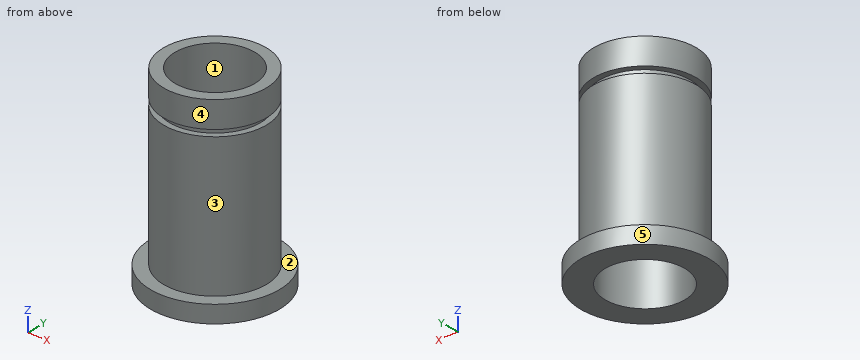
```python
from build123d import *


with BuildPart() as part:
    # Sketch1 → Revolve1 (revolve)
    with BuildSketch(Plane(origin=(0, 0, 0), x_dir=(0, 0, -1), z_dir=(1, 0, 0)), mode=Mode.PRIVATE) as revolve1_sk:
        Polygon((0, 5.9182), (3.048, 5.9182), (3.048, 5.2324), (3.7846, 5.2324), (3.7846, 5.9182), (20, 5.9182), (20, 7.4182), (22, 7.4182), (22, 4.6), (0, 4.6), align=None)
    revolve(revolve1_sk.sketch.rotate(Axis((0, 0, 0), (0, 0, -1)), 90), axis=Axis((0, 0, 0), (0, 0, -1)))  # turned: the seam where the file's is


solid = part.part
```
Input: part model. Units: mm. Frame: model coordinates. Face numbers are marked on the shaded views. A direction names the side the tool comes from. Round coordinates to 2 decimals unless told otherwise and drop trailing zeros. Write each loop counter-clockwise with the first axis right and the second up, starting at its lowest first coordinate (ties: lowest second). Pieces come first, ordered by that corner, then holes. Notation, with made-up numbers: (84.5, 69.25) -> (106.5, 69.25) arc R23 cw to (106.5, 86.25) -> close; hole circle Ø10 at (68, 85.25). An arc over 180 degrees is marked (long way). Answer as CSV lines item,"result".
1. Mould query, pull axis Y, two halves, no side actions, for the marked faces 1, 2 and 3. Classes: +Y half, -Y half, draft (parallel to the pull), parting line (faces both ways), or undercut.
Geometry says:
face 1,"undercut"
face 2,"draft"
face 3,"parting line"
2. Section C-C (z = -19.5). Return the cut outline in (x, y).
Geometry says:
outline,"circle Ø11.84 at (0, 0); hole circle Ø9.2 at (0, 0)"
3. Contact query for flat-ended pins moving along their axis: P1, Ø5, axis at x = -0.5, z = -13.5, coming from the -Y side; P2, Ø3, axis at y = -3, z = -10, coming from the +X side; P3, Ø6, axis at x = -4, z = -18.5, coming from the -Y side. Output: stop coordinate, or through.
Geometry says:
P1,"stops at y = -5.92"
P2,"stops at x = 5.72"
P3,"stops at y = -7.28"
4. Reachability of the marked faces 4 and 5 from +Z, -Z, +X, -X, +Y, -Y: full face, straight path, thin tool, end or side. Return the list, or none.
Geometry says:
face 4,"+Z"
face 5,"+Z, -Z"
5. Section A-A (y = 0). Return the cut outline in (x, z), plus the area to 3 significant figures.
Geometry says:
outline,"(-7.42, -22) -> (-4.6, -22) -> (-4.6, 0) -> (-5.92, 0) -> (-5.92, -3.05) -> (-5.23, -3.05) -> (-5.23, -3.78) -> (-5.92, -3.78) -> (-5.92, -20) -> (-7.42, -20) -> close; (4.6, -22) -> (7.42, -22) -> (7.42, -20) -> (5.92, -20) -> (5.92, -3.78) -> (5.23, -3.78) -> (5.23, -3.05) -> (5.92, -3.05) -> (5.92, 0) -> (4.6, 0) -> close"
area,"63.0 mm^2"
6. Ray query, L1, parallel to Z at x = -5.25, y = -2.25; L2, parallel to Y at x = 0, z = -14.5; L3, parallel to Z at x = -5.5, y = 3. Return the intervals inside material, ascending. Write a range as [from, to].
Geometry says:
L1,"z = [-22, -3.78], [-3.05, 0]"
L2,"y = [-5.92, -4.6], [4.6, 5.92]"
L3,"z = [-22, -20]"
